```python
from build123d import *

# Parameters (mm, degrees)
PAD_DEPTH         = 10
SKETCH001_R       = 1.6
POCKET_DEPTH      = 19.001
SKETCH003_R       = 3.75
SKETCH003_R_2     = 1.6
PAD001_DEPTH      = 17
PAD001_FACE15_R   = 3.75
PAD001_FACE15_R_2 = 1.6
POCKET001_DEPTH   = 8
FILLET_R          = 4.999
FILLET_FACE4_W    = 2
FILLET_FACE4_H    = 10
POCKET002_DEPTH   = 1
FILLET001_R       = 2


with BuildPart() as part:
    # Sketch → Pad (new body)
    with BuildSketch(Plane.XY):
        Polygon((-19.5, -1), (-19.5, 18), (-9.5, 18), (7.264706, 3), (7.264706, 1), (-9.5, 1), (-9.5, -1), align=None)
    extrude(amount=PAD_DEPTH)

    # Sketch001 (on Face3 of Pad) → Pocket (cut, through all)
    with BuildSketch(Plane.XZ.offset(1)):
        with Locations((-14.5, 5)):
            Circle(SKETCH001_R)
        with Locations((-1.117647, 5)):
            Circle(SKETCH001_R)
    extrude(amount=-POCKET_DEPTH, mode=Mode.SUBTRACT)

    # Sketch003 (on Face1 of Pocket) → Pad001 (join)
    with BuildSketch(Plane.XZ.offset(-1)):
        with Locations((-1.117647, 5)):
            Circle(SKETCH003_R)
        with Locations((-1.117647, 5)):
            Circle(SKETCH003_R_2, mode=Mode.SUBTRACT)
    extrude(amount=-PAD001_DEPTH)

    # Pad001 Face15 → Pocket001 (cut)
    with BuildSketch(Plane(origin=(-1.117647, 18, 5), x_dir=(1, 0, 0), z_dir=(0, 1, 0))):
        Circle(PAD001_FACE15_R)
        Circle(PAD001_FACE15_R_2, mode=Mode.SUBTRACT)
    extrude(amount=-POCKET001_DEPTH, mode=Mode.SUBTRACT)

    # Fillet
    fillet_edges = [part.edges().sort_by_distance(p)[0] for p in [
        (-19.5, 8.5, 10),
        (-19.5, 8.5, 0),
        (7.264706, 2, 10),
        (7.264706, 2, 0),
    ]]
    fillet(fillet_edges, radius=FILLET_R)

    # Fillet Face4 → Pocket002 (cut)
    with BuildSketch(Plane(origin=(-9.5, 0, 5), x_dir=(0, -1, 0), z_dir=(1, 0, 0))):
        Rectangle(FILLET_FACE4_W, FILLET_FACE4_H)
    extrude(amount=-POCKET002_DEPTH, mode=Mode.SUBTRACT)

    # Fillet001
    fillet001_edges = [part.edges().sort_by_distance(p)[0] for p in [
        (-10.5, 0, 0),
        (-10.5, 0, 10),
    ]]
    fillet(fillet001_edges, radius=FILLET001_R)


solid = part.part
```
The model under review builds one solid part; all positions refer to its coordinate system, in mm. A direction names the side the tool comes from. Give positions to 0.01 mm unless a question says otherwise; leave off trailing zeros. Loops run counter-clockwise (first coordinate to the right, second up) from the corner with the lowest first, then second, coordinate; pieces in that order, holes last. Notation, with made-up numbers: (86, 44) -> (132, 44) arc R14 ccw to (132, 55) -> close; hole circle Ø1 at (6, 83). An arc over 180 degrees is marked (long way). Use CSV: the item, a comma, the result in double quotes.
1. Consider section C-C, the plane z = 2.5. Write out the cut boundary in (x, y), then the cut area to 3 significant figures.
Result:
outline,"(-18.83, -1) -> (-10.5, -1) -> (-10.5, 1) -> (6.6, 1) -> (6.6, 3.6) -> (1.68, 8) -> (1.68, 10) -> (-3.91, 10) -> (-3.91, 13) -> (-9.5, 18) -> (-18.83, 18) -> close"
area,"330 mm²"
2. For P1, Ø6, axis at x = -1.12, z = 5, coming from the +Y side; P2, Ø5, axis at x = -6.5, z = 3.5, coming from the +Y side; P3, Ø5, axis at x = -3, z = 4.5, coming from the -Y side, all flat-tipped, find the tip position at first contact; note any pin that passes through.
Result:
P1,"stops at y = 10"
P2,"stops at y = 17.55"
P3,"stops at y = 1"
3. Consider section D-D, the plane x = -7. Write out the cut boundary in (y, z), then the cut area to 3 significant figures.
Result:
outline,"(1, 0) -> (15.76, 0) -> (15.76, 10) -> (1, 10) -> close"
area,"148 mm²"
4. Consider section A-A, the plane z = 4.25. Write out the cut boundary in (x, y).
Result:
outline,"(-19.44, -1) -> (-15.91, -1) -> (-15.91, 18) -> (-19.44, 18) -> close; (-13.09, -1) -> (-10.5, -1) -> (-10.5, 1) -> (-2.53, 1) -> (-2.53, 10) -> (-4.79, 10) -> (-4.79, 13.79) -> (-9.5, 18) -> (-13.09, 18) -> close; (0.3, 1) -> (7.21, 1) -> (7.21, 3.05) -> (2.56, 7.21) -> (2.56, 10) -> (0.3, 10) -> close"
5. To check wall thickness, follow probe 1 along Z at (x, y) = (-14.5, 6.25); probe 2 along X at (y, z) = (8, 3.75); probe 3 along X at (y, z) = (13, 6). State the ranges of each line that lie inside material, in increasing order. Write a range as from..to.
Result:
probe 1,"z = 0..3.4, 6.6..10"
probe 2,"x = -19.34..-15.5, -13.5..-2.12, -0.12..2.42"
probe 3,"x = -19.4..-15.75, -13.25..-4.73"
6. Machinability: for faces 4 (the face through (-11.1, -0.01, 0.57)), 5 (the face through (-11.07, -0.01, 9.4)), 6 (the face through (2.63, 8.87, 4.93)), 7 (the face through (-10.5, 0, 5)), which of the approach directions +Z, -Z, +X, -X, +Y, -Y give a long, thin tool a straight path to every point of the face, cutting with its end or side? Answer none if there is none.
Result:
face 4,"-Z, +X, -Y"
face 5,"+Z, +X, -Y"
face 6,"+X, +Y"
face 7,"+Z, -Z, +X, -Y"
7. Consider section B-B, the plane y = 4.5. Count the separate pieces of the cut face and the enclosed holes in it, then the cut area to 3 significant figures.
Result:
separate pieces,"1"
enclosed holes,"2"
area,"221 mm²"
8. The part is to be moulded in two halves that separate along X. For faces 1 (the face through (-3.098, 12.272, 1.597)), 2 (the face through (-8, 9, 10)), 3 (the face through (-1.464, 5.437, 3.438)), say which applies: +X half, -X half, draft (parallel to the pull), parting line (faces both ways), or undercut.
Result:
face 1,"+X half"
face 2,"draft"
face 3,"undercut"
